Source: three-view drawing plus pictorial views. Frame: mm from the lowest corner of the part. A direction names the side the tool comes from. Give positions to 0.01 mm unless a question says otherwise; leave off trailing zeros. Order: outer loops, then holes, each group sorted by start corner. A loop starts at its lowest first (then second) coordinate and runs counter-clockwise, first axis right, second up. Notation, with made-up numbers: (82, 50.5) -> (125, 50.5) arc R4 cw to (125, 54.5) -> close; hole circle Ø5 at (67, 89.5). An arc over 180 degrees is marked (long way). Answer in a Markdown table with one row per item.
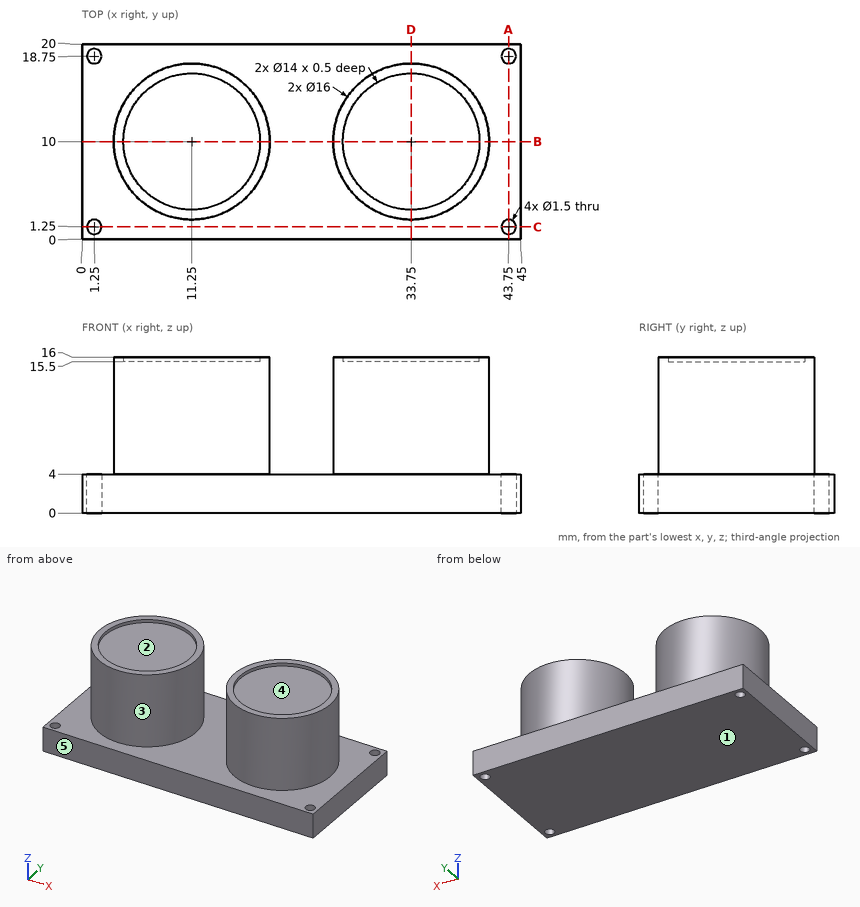
(1) Section query A-A (x = 43.75). Return the cut outline in (y, z), plus the area to 3 significant figures.
A:
| item | result |
|---|---|
| outline | (0, 0) -> (0.5, 0) -> (0.5, 4) -> (0, 4) -> close; (2, 0) -> (18, 0) -> (18, 4) -> (2, 4) -> close; (19.5, 0) -> (20, 0) -> (20, 4) -> (19.5, 4) -> close |
| area | 68.0 mm^2 |
(2) First-contact query: pin 1 Ø1 at (x, z) = (12, 8.5) entering from -Y; pin 2 Ø2.5 at (x, y) = (1.25, 1.25) entering from +Z; pin 3 Ø4 at (x, y) = (31, 8) entering from +Z. Flat tips, straight axial feed; report the tip coordinate or a pass-through.
A:
| item | result |
|---|---|
| pin 1 | stops at y = 2 |
| pin 2 | stops at z = 4 |
| pin 3 | stops at z = 15.5 |
(3) Access query for the marked faces 1 and 2. Directions: +Z, -Z, +X, -X, +Y, -Y. A direction counts if a zero-diameter tool reaches every point of the face in a straight line with its end or side. Return the directions, or none.
A:
| item | result |
|---|---|
| face 1 | -Z, +X, -X, +Y, -Y |
| face 2 | +Z |
(4) Pull-direction query (Y, two-part tool) for the marked faces 3, 4 and 5; classes: +Y half, -Y half, draft (parallel to the pull), parting line (faces both ways), or undercut.
A:
| item | result |
|---|---|
| face 3 | parting line |
| face 4 | undercut |
| face 5 | -Y half |
(5) Section query C-C (y = 1.25). Return the cut outline in (x, z).
A:
| item | result |
|---|---|
| outline | (0, 0) -> (0.5, 0) -> (0.5, 4) -> (0, 4) -> close; (2, 0) -> (43, 0) -> (43, 4) -> (2, 4) -> close; (44.5, 0) -> (45, 0) -> (45, 4) -> (44.5, 4) -> close |
(6) Section query D-D (x = 33.75). Return the cut outline in (y, z), plus the area to 3 significant figures.
A:
| item | result |
|---|---|
| outline | (0, 0) -> (20, 0) -> (20, 4) -> (18, 4) -> (18, 16) -> (17, 16) -> (17, 15.5) -> (3, 15.5) -> (3, 16) -> (2, 16) -> (2, 4) -> (0, 4) -> close |
| area | 265 mm^2 |
(7) Ray query, probe 1 along Y at (x, z) = (1.25, 2.35); probe 2 along X at (y, z) = (10, 15.7); probe 3 along X at (y, z) = (10, 12.25). Return the intervals inside material, ascending.
A:
| item | result |
|---|---|
| probe 1 | y = 0 to 0.5, 2 to 18, 19.5 to 20 |
| probe 2 | x = 3.25 to 4.25, 18.25 to 19.25, 25.75 to 26.75, 40.75 to 41.75 |
| probe 3 | x = 3.25 to 19.25, 25.75 to 41.75 |
(8) Section query B-B (y = 10). Return the cut outline in (x, z).
A:
| item | result |
|---|---|
| outline | (0, 0) -> (45, 0) -> (45, 4) -> (41.75, 4) -> (41.75, 16) -> (40.75, 16) -> (40.75, 15.5) -> (26.75, 15.5) -> (26.75, 16) -> (25.75, 16) -> (25.75, 4) -> (19.25, 4) -> (19.25, 16) -> (18.25, 16) -> (18.25, 15.5) -> (4.25, 15.5) -> (4.25, 16) -> (3.25, 16) -> (3.25, 4) -> (0, 4) -> close |
